Could you check a few things on this model? Use its own coordinates, in mm. A direction names the side the tool comes from. Coordinates: 2 decimals unless noted, no trailing zeros. Loops run counter-clockwise (first coordinate to the right, second up) from the corner with the lowest first, then second, coordinate; pieces in that order, holes last.
1) If I drill on line 1 along Y through (x, z) = (0, 4.5); line 2 along X through (y, z) = (-0.5, 1.75) (3 decimals); line 3 along Y through (x, z) = (3.75, 6), over which ranges is the centre line in solid material (lowest first)?
2) Imagine slicing it at A-A on x = 0. Please give me the cut outline in (y, z), plus the area to 3 significant figures.
3) Thinking about a two-plate mould opening in X: for faces 1 (the face through (0, 4.762, 3)), 2 (the face through (4.73, 2.51, 2.33)), 3 (the face through (9.525, 3, 3)), which applies, released by +X, released by -X, zero draft, split by the parting line, or undercut?
4) Will this pin go through, and if not, where does the flat tip stop? P1, Ø3.5, axis at x = -6.35, z = 3.175, coming from the +Y side.
5) Imagine slicing it at B-B on z = 2.75. Please give me the cut outline in (x, y) (1 decimal), plus the area to 3 significant figures.
6) Imagine slicing it at D-D on y = 2. Please give me the cut outline in (x, z) (3 decimals), plus the area to 4 significant figures.
7) For faces 4 (the face through (4, 0.318, 3)), 5 (the face through (-8.135, -0.067, 3.571)), which set-ups out of +Z, -Z, +X, -X, +Y, -Y let a thin tool reach every point of the face, with its end or its side?
```python
from build123d import *

# Parameters (mm, degrees)
BOSS_EXTRUDE1_DEPTH = 6.35
SKETCH2_R           = 1.8288
CUT_EXTRUDE1_DEPTH  = 15.892070037


with BuildPart() as part:
    # Sketch1 → Boss-Extrude1 (new body)
    with BuildSketch(Plane.XY):
        with BuildLine():
            Line((-9.525, -4.7625), (9.525, -4.7625))
            Line((9.525, -4.7625), (9.525, -0.3175))
            Line((9.525, -0.3175), (1.555425987, -0.3175))
            ThreePointArc((1.555425987, -0.3175), (-1.5875, 0), (1.555425987, 0.3175))
            Line((1.555425987, 0.3175), (9.525, 0.3175))
            Line((9.525, 0.3175), (9.525, 4.7625))
            Line((9.525, 4.7625), (-9.525, 4.7625))
            Line((-9.525, 4.7625), (-9.525, -4.7625))
        make_face()
    extrude(amount=BOSS_EXTRUDE1_DEPTH)

    # Sketch2 → Cut-Extrude1 (cut, through all)
    with BuildSketch(Plane.XZ.offset(4.7625)):
        with Locations(Location((-6.35, 3.175, 0), (0, 0, 270))):
            Circle(SKETCH2_R)
        with Locations(Location((6.35, 3.175, 0), (0, 0, 270))):
            Circle(SKETCH2_R)
    extrude(amount=-CUT_EXTRUDE1_DEPTH, mode=Mode.SUBTRACT)


solid = part.part
```
Filled in:
1. line 1: y = -4.76 to -1.59, 1.59 to 4.76
1. line 2: x = -9.525 to -7.496, -5.204 to -1.507, 1.507 to 5.204, 7.496 to 9.525
1. line 3: y = -4.76 to -0.32, 0.32 to 4.76
2. outline: (-4.76, 0) - (-1.59, 0) - (-1.59, 6.35) - (-4.76, 6.35) - close; (1.59, 0) - (4.76, 0) - (4.76, 6.35) - (1.59, 6.35) - close
2. area: 40.3 mm2
3. face 1: zero draft
3. face 2: undercut
3. face 3: released by +X
4. P1: passes through
5. outline: (-9.5, -4.8) - (-8.1, -4.8) - (-8.1, 4.8) - (-9.5, 4.8) - close; (-4.6, -4.8) - (4.6, -4.8) - (4.6, -0.3) - (1.6, -0.3) arc R1.6 cw (long way) to (1.6, 0.3) - (4.6, 0.3) - (4.6, 4.8) - (-4.6, 4.8) - close; (8.1, -4.8) - (9.5, -4.8) - (9.5, -0.3) - (8.1, -0.3) - close; (8.1, 0.3) - (9.5, 0.3) - (9.5, 4.8) - (8.1, 4.8) - close
5. area: 103 mm2
6. outline: (-9.525, 0) - (9.525, 0) - (9.525, 6.35) - (-9.525, 6.35) - close; hole circle Ø3.658 at (-6.35, 3.175); hole circle Ø3.658 at (6.35, 3.175)
6. area: 100.0 mm2
7. face 4: +Z, -Z, +X
7. face 5: +Y, -Y
